The drawing under review shows one solid part. Ordinate dimensions are in mm from its lowest x, y, z. Give positions to 0.01 mm unless a question says otherwise; leave off trailing zeros. Write each loop counter-clockwise with the first axis right and the second up, starting at its lowest first coordinate (ties: lowest second). Pieces come first, ordered by that corner, then holes. Notation, with made-up numbers: (-12, 24) -> (33, 24) arc R5 cw to (33, 32) -> close; hole circle Ø7 at (52.25, -31). An arc over 180 degrees is marked (long way). Put each result on its own line as item: value. Start each with the question number.
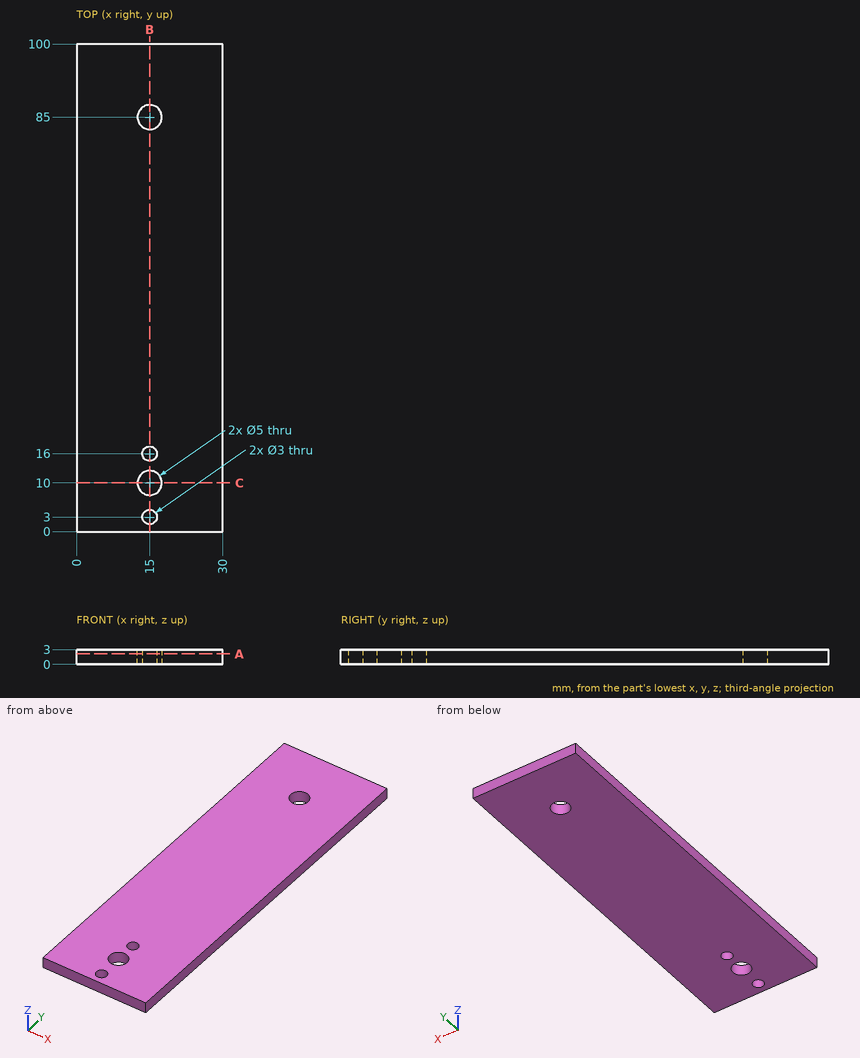
Q1. Take a section at A-A on z = 2.15. Give the boundary of the cut face in (x, y), then the cut area to 3 significant figures.
Q2. For pin 1 (4 mm diameter, centred on x = 15, y = 85, fed in from +Z), flat-tipped, find the tip position at first contact; note if it passes through.
Q3. Take a section at B-B on x = 15. Give the boundary of the cut face in (y, z), then the cut area to 3 significant figures.
Q4. Take a section at C-C on y = 10. Give the boundary of the cut face in (x, z), then the cut area to 3 significant figures.
Q5. To check wall thickness, follow probe 1 along Y at (x, z) = (15, 2.15); probe 2 along X at (y, z) = (3, 1.85); probe 3 along X at (y, z) = (10.5, 0.35). State the ranges of each line that lie inside material, in increasing order. Write a range as from..to.
Result:
1. outline: (0, 0) -> (30, 0) -> (30, 100) -> (0, 100) -> close; hole circle Ø5 at (15, 10); hole circle Ø5 at (15, 85); hole circle Ø3 at (15, 3); hole circle Ø3 at (15, 16)
1. area: 2,950 mm^2
2. pin 1: passes through
3. outline: (0, 0) -> (1.5, 0) -> (1.5, 3) -> (0, 3) -> close; (4.5, 0) -> (7.5, 0) -> (7.5, 3) -> (4.5, 3) -> close; (12.5, 0) -> (14.5, 0) -> (14.5, 3) -> (12.5, 3) -> close; (17.5, 0) -> (82.5, 0) -> (82.5, 3) -> (17.5, 3) -> close; (87.5, 0) -> (100, 0) -> (100, 3) -> (87.5, 3) -> close
3. area: 252 mm^2
4. outline: (0, 0) -> (12.5, 0) -> (12.5, 3) -> (0, 3) -> close; (17.5, 0) -> (30, 0) -> (30, 3) -> (17.5, 3) -> close
4. area: 75.0 mm^2
5. probe 1: y = 0..1.5, 4.5..7.5, 12.5..14.5, 17.5..82.5, 87.5..100
5. probe 2: x = 0..13.5, 16.5..30
5. probe 3: x = 0..12.55, 17.45..30
